```python
from build123d import *

# Parameters (mm, degrees)
F0_W       = 228.6
F0_H       = 127
F0_R       = 4.7625
F1_DEPTH   = 12.7
F2_W       = 12.7
F2_H       = 127
F3_DEPTH   = 12.7
F4_W       = 228.6
F4_H       = 12.7
F5_DEPTH   = 9.525
F6_SIZE2   = 19.05
F6_SIZE    = 6.35
F7_R       = 3.175
F8_R       = 3.175
F9_SIZE2   = 6.35
F9_SIZE    = 19.05
F9_2_SIZE2 = 6.35
F9_2_SIZE  = 19.05
F10_R      = 3.175
F11_R      = 3.175


with BuildPart() as f1:
    # F0 (on Top) → F1 (new body)
    with BuildSketch(Plane.XY):
        Rectangle(F0_W, F0_H)
        with Locations((-101.6, -50.8)):
            Circle(F0_R, mode=Mode.SUBTRACT)
        with Locations((101.6, -50.8)):
            Circle(F0_R, mode=Mode.SUBTRACT)
        with Locations((-101.6, 50.8)):
            Circle(F0_R, mode=Mode.SUBTRACT)
        with Locations((101.6, 50.8)):
            Circle(F0_R, mode=Mode.SUBTRACT)
    extrude(amount=F1_DEPTH)

    # F2 (on face) → F3 (join)
    with BuildSketch(Plane(origin=(0, 0, 0), x_dir=(1, 0, 0), z_dir=(0, 0, -1))):
        with Locations((-82.55, 0)):
            Rectangle(F2_W, F2_H)
        with Locations((82.55, 0)):
            Rectangle(F2_W, F2_H)
    extrude(amount=F3_DEPTH)

    # F4 (on face) → F5 (join)
    with BuildSketch(Plane(origin=(0, 0, 0), x_dir=(1, 0, 0), z_dir=(0, 0, -1))):
        with Locations((0, -31.75)):
            Rectangle(F4_W, F4_H)
        with Locations((0, 31.75)):
            Rectangle(F4_W, F4_H)
    extrude(amount=F5_DEPTH)

    # F6
    f6_edges = [f1.edges().sort_by_distance(p)[0] for p in [
        (-114.3, -31.75, -9.525),
        (-114.3, 31.75, -9.525),
    ]]
    f6_side = f1.faces().sort_by_distance((-114.3, 0, 4.900543))[0]
    chamfer(f6_edges, length=F6_SIZE, length2=F6_SIZE2, reference=f6_side)

    # F7
    f7_edges = [f1.edges().sort_by_distance(p)[0] for p in [
        (-114.3, -31.75, -3.175),
        (-114.3, 31.75, -3.175),
        (-95.25, -31.75, -9.525),
        (-95.25, 31.75, -9.525),
    ]]
    fillet(f7_edges, radius=F7_R)

    # F8
    f8_edges = [f1.edges().sort_by_distance(p)[0] for p in [
        (-82.55, -63.5, -12.7),
        (-82.55, 63.5, -12.7),
        (82.55, 63.5, -12.7),
        (82.55, -63.5, -12.7),
    ]]
    fillet(f8_edges, radius=F8_R)

    # F9
    f9_edges = [f1.edges().sort_by_distance(p)[0] for p in [
        (114.3, -31.75, -9.525),
    ]]
    f9_side = f1.faces().sort_by_distance((101.6, -31.75, -9.525))[0]
    chamfer(f9_edges, length=F9_SIZE, length2=F9_SIZE2, reference=f9_side)

    # F9#2
    f9_2_edges = [f1.edges().sort_by_distance(p)[0] for p in [
        (114.3, 31.75, -9.525),
    ]]
    f9_2_side = f1.faces().sort_by_distance((101.6, 31.75, -9.525))[0]
    chamfer(f9_2_edges, length=F9_2_SIZE, length2=F9_2_SIZE2, reference=f9_2_side)

    # F10
    f10_edges = [f1.edges().sort_by_distance(p)[0] for p in [
        (114.3, -31.75, -3.175),
        (114.3, 31.75, -3.175),
        (95.25, 31.75, -9.525),
        (95.25, -31.75, -9.525),
    ]]
    fillet(f10_edges, radius=F10_R)

    # F11
    f11_edges = [f1.edges().sort_by_distance(p)[0] for p in [
        (-114.3, -63.5, 6.35),
        (-114.3, 63.5, 6.35),
        (114.3, -63.5, 6.35),
        (114.3, 63.5, 6.35),
    ]]
    fillet(f11_edges, radius=F11_R)


solid = f1.part
```
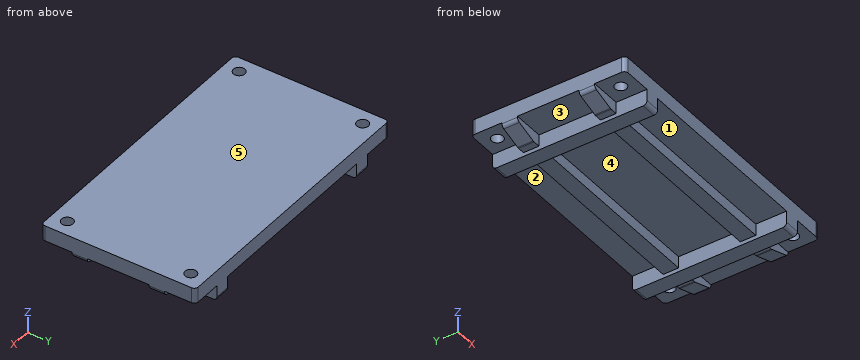
Build history of the part. All positions in model axes, mm. Face numbers are marked on the shaded views. A direction names the side the tool comes from. Round coordinates to 2 decimals unless told otherwise and drop trailing zeros. Write each loop counter-clockwise with the first axis right and the second up, starting at its lowest first coordinate (ties: lowest second). Pieces come first, ordered by that corner, then holes. Notation, with made-up numbers: (54.5, -39) -> (102.5, -39) arc R21 cw to (102.5, -1) -> close; hole circle Ø9 at (17.5, -7.75). An arc over 180 degrees is marked (long way). Put each result on its own line as item: value.
Item 1: Two-plate mould, pull along Y, no slides. Class the marked faces 3, 4 and 5: pulls with the +Y half, pulls with the -Y half, needs draft (parallel to the pull), parting line crosses it, or undercut.
Here are the results:
face 3: undercut
face 4: undercut
face 5: needs draft
Item 2: Slice it at C-C, the plane x = 13.5. Give the cut face in (y, z) (3 decimals).
Here are the results:
outline: (-63.5, 0) -> (-38.1, 0) -> (-38.1, -9.525) -> (-25.4, -9.525) -> (-25.4, 0) -> (25.4, 0) -> (25.4, -9.525) -> (38.1, -9.525) -> (38.1, 0) -> (63.5, 0) -> (63.5, 12.7) -> (-63.5, 12.7) -> close
Item 3: Slice it at B-B, the plane y = -50.8. Give the cut face in (x, z).
Here are the results:
outline: (-114.3, 0) -> (-106.36, 0) -> (-106.36, 12.7) -> (-114.3, 12.7) -> close; (-96.84, 0) -> (-88.9, 0) -> (-88.9, -12.7) -> (-76.2, -12.7) -> (-76.2, 0) -> (76.2, 0) -> (76.2, -12.7) -> (88.9, -12.7) -> (88.9, 0) -> (96.84, 0) -> (96.84, 12.7) -> (-96.84, 12.7) -> close; (106.36, 0) -> (114.3, 0) -> (114.3, 12.7) -> (106.36, 12.7) -> close
Item 4: Slice it at A-A, the plane x = -101.6. Give the cut face in (y, z), plus the area to 3 significant figures.
Here are the results:
outline: (-63.5, 0) -> (-55.56, 0) -> (-55.56, 12.7) -> (-63.5, 12.7) -> close; (-46.04, 0) -> (-38.1, 0) -> (-38.1, -7.41) -> (-25.4, -7.41) -> (-25.4, 0) -> (25.4, 0) -> (25.4, -7.41) -> (38.1, -7.41) -> (38.1, 0) -> (46.04, 0) -> (46.04, 12.7) -> (-46.04, 12.7) -> close; (55.56, 0) -> (63.5, 0) -> (63.5, 12.7) -> (55.56, 12.7) -> close
area: 1,560 mm^2
Item 5: Wall check: probe 1 along Y at (x, z) = (-101.6, 7.5); probe 2 along X at (y, z) = (18, -0.75); probe 3 along Y at (x, z) = (-94, -1.25). Give the ranges that are in metal, low to high. Write a range as from..to.
Here are the results:
probe 1: y = -63.5..-55.56, -46.04..46.04, 55.56..63.5
probe 2: x = -88.9..-76.2, 76.2..88.9
probe 3: y = -38.1..-25.4, 25.4..38.1
Item 6: Flat gauge pins, fed straight in: P1, Ø14, axis at y = 11, z = -7.5, coming from the -X side; P2, Ø4, axis at x = -28.5, z = -3, coming from the +Y side; P3, Ø11, axis at x = -101.6, y = -50.8, coming from the -Z side. Where does each tip first touch, or does it go through?
Here are the results:
P1: stops at x = -88.9
P2: stops at y = 38.1
P3: stops at z = 0
Item 7: Tool access for the marked faces 1 and 2: list every direction of +Z, -Z, +X, -X, +Y, -Y with a clear straight run to the whole face (end or side of a thin tool).
Here are the results:
face 1: -Z, -Y
face 2: -Z, +Y
